from build123d import *

# Parameters (mm, degrees)
SKETCH1_W           = 50
SKETCH1_H           = 40
SKETCH1_W_2         = 44
SKETCH1_H_2         = 35.2
BOSS_EXTRUDE1_DEPTH = 5
SKETCH2_W           = 44
SKETCH2_H           = 35.2
BOSS_EXTRUDE2_DEPTH = 3
SKETCH3_R           = 6
BOSS_EXTRUDE3_DEPTH = 2
SKETCH4_R           = 1.6
CUT_EXTRUDE1_DEPTH  = 5
FILLET1_R           = 6
FILLET2_R           = 3
CUT_EXTRUDE2_DEPTH  = 3
SKETCH8_R           = 4
CUT_EXTRUDE3_DEPTH  = 3
CHAMFER1_SIZE       = 1
SKETCH9_W           = 3
SKETCH9_H           = 15
CUT_EXTRUDE4_DEPTH  = 2
FILLET3_R           = 2
BOSS_EXTRUDE5_START = 4
BOSS_EXTRUDE5_DEPTH = 4
SKETCH11_R          = 4
CUT_EXTRUDE5_DEPTH  = 4


with BuildPart() as part:
    # Sketch1 → Boss-Extrude1 (new body)
    with BuildSketch(Plane(origin=(0, 0, 0), x_dir=(1, 0, 0), z_dir=(0, 1, 0))):
        Rectangle(SKETCH1_W, SKETCH1_H)
        Rectangle(SKETCH1_W_2, SKETCH1_H_2, mode=Mode.SUBTRACT)
    extrude(amount=BOSS_EXTRUDE1_DEPTH)

    # Sketch2 → Boss-Extrude2 (add)
    with BuildSketch(Plane(origin=(0, 0, 0), x_dir=(-1, 0, 0), z_dir=(0, -1, 0))):
        Rectangle(SKETCH2_W, SKETCH2_H)
    extrude(amount=-BOSS_EXTRUDE2_DEPTH)

    # Sketch3 → Boss-Extrude3 (add)
    with BuildSketch(Plane(origin=(0, 3, 0), x_dir=(1, 0, 0), z_dir=(0, 1, 0))):
        with Locations(Location((7, 0, 0), (0, 0, 270))):
            Circle(SKETCH3_R)
    extrude(amount=BOSS_EXTRUDE3_DEPTH)

    # Sketch4 → Cut-Extrude1 (cut)
    with BuildSketch(Plane(origin=(0, 5, 0), x_dir=(1, 0, 0), z_dir=(0, 1, 0))):
        with Locations(Location((7, 0, 0), (0, 0, 270))):
            Circle(SKETCH4_R)
    extrude(amount=-CUT_EXTRUDE1_DEPTH, mode=Mode.SUBTRACT)

    # Fillet1
    fillet1_edges = [part.edges().sort_by_distance(p)[0] for p in [
        (22, 4, 17.6),
        (22, 4, -17.6),
        (-22, 4, -17.6),
        (-22, 4, 17.6),
        (-25, 2.5, -20),
        (25, 2.5, -20),
        (25, 2.5, 20),
        (-25, 2.5, 20),
    ]]
    fillet(fillet1_edges, radius=FILLET1_R)

    # Fillet2
    fillet2_edges = [part.edges().sort_by_distance(p)[0] for p in [
        (-25, 0, 0),
        (0, 0, -20),
        (25, 0, 0),
        (0, 0, 20),
        (23.242640687, 0, -18.242640687),
        (23.242640687, 0, 18.242640687),
        (-23.242640687, 0, 18.242640687),
        (-23.242640687, 0, -18.242640687),
    ]]
    fillet(fillet2_edges, radius=FILLET2_R)

    # Sketch6 → Cut-Extrude2 (cut)
    with BuildSketch(Plane(origin=(0, 0, 0), x_dir=(-1, 0, 0), z_dir=(0, -1, 0))):
        Polygon((-3.75, 0), (-5.375, 2.814582562), (-8.625, 2.814582562), (-10.25, 0), (-8.625, -2.814582562), (-5.375, -2.814582562), align=None)
    extrude(amount=-CUT_EXTRUDE2_DEPTH, mode=Mode.SUBTRACT)

    # Sketch8 → Cut-Extrude3 (cut)
    with BuildSketch(Plane(origin=(0, 0, 0), x_dir=(-1, 0, 0), z_dir=(0, -1, 0))):
        with Locations(Location((-12, -10, 0), (0, 0, 90))):
            Circle(SKETCH8_R)
        with Locations(Location((-12, 10, 0), (0, 0, 90))):
            Circle(SKETCH8_R)
    extrude(amount=-CUT_EXTRUDE3_DEPTH, mode=Mode.SUBTRACT)

    # Chamfer1
    chamfer1_edges = [part.edges().sort_by_distance(p)[0] for p in [
        (12, 0, 14),
        (12, 0, -6),
    ]]
    chamfer(chamfer1_edges, length=CHAMFER1_SIZE)

    # Sketch9 → Cut-Extrude4 (cut)
    with BuildSketch(Plane(origin=(0, 5, 0), x_dir=(1, 0, 0), z_dir=(0, 1, 0))):
        with Locations((23.5, 0)):
            Rectangle(SKETCH9_W, SKETCH9_H)
    extrude(amount=-CUT_EXTRUDE4_DEPTH, mode=Mode.SUBTRACT)

    # Fillet3
    fillet3_edges = [part.edges().sort_by_distance(p)[0] for p in [
        (23.5, 3, -7.5),
        (23.5, 3, 7.5),
    ]]
    fillet(fillet3_edges, radius=FILLET3_R - 0.0001)  # a hair under: the kernel refuses the full size

    # Sketch10 → Boss-Extrude5 (add)
    with BuildSketch(Plane(origin=(0, 3, 0), x_dir=(1, 0, 0), z_dir=(0, 1, 0)).offset(BOSS_EXTRUDE5_START)):
        with BuildLine():
            Line((-16, -17.6), (-16, -11.6))
            Line((-16, -11.6), (-22, -11.6))
            ThreePointArc((-22, -11.6), (-20.242640687, -15.842640687), (-16, -17.6))
        make_face()
        with BuildLine():
            Line((-16, 17.6), (-16, 11.6))
            Line((-16, 11.6), (-22, 11.6))
            ThreePointArc((-22, 11.6), (-20.242640687, 15.842640687), (-16, 17.6))
        make_face()
        with BuildLine():
            Line((16, 17.6), (16, 11.6))
            Line((16, 11.6), (22, 11.6))
            ThreePointArc((22, 11.6), (20.242640687, 15.842640687), (16, 17.6))
        make_face()
        with BuildLine():
            Line((22, -11.6), (16, -11.6))
            Line((16, -11.6), (16, -17.6))
            ThreePointArc((16, -17.6), (20.242640687, -15.842640687), (22, -11.6))
        make_face()
    extrude(amount=-BOSS_EXTRUDE5_DEPTH)

    # Sketch11 → Cut-Extrude5 (cut)
    with BuildSketch(Plane(origin=(0, 7, 0), x_dir=(1, 0, 0), z_dir=(0, 1, 0))):
        with Locations((16, 11.6)):
            Circle(SKETCH11_R)
        with Locations((16, -11.6)):
            Circle(SKETCH11_R)
        with Locations((-16, -11.6)):
            Circle(SKETCH11_R)
        with Locations((-16, 11.6)):
            Circle(SKETCH11_R)
    extrude(amount=-CUT_EXTRUDE5_DEPTH, mode=Mode.SUBTRACT)


solid = part.part
Can you work these out from the model? Positions are in its coordinate system, mm. A direction names the side the tool comes from. Give positions to 0.01 mm unless a question says otherwise; leave off trailing zeros. Loops run counter-clockwise (first coordinate to the right, second up) from the corner with the lowest first, then second, coordinate; pieces in that order, holes last. Notation, with made-up numbers: M 51.5,70.5 L 90.5,70.5 A24 cw 90.5,84.5 Z; hole C 9,46.5 d7. An arc over 180 degrees is marked long. One line per item, written item: value. Start each with the question number.
1) If we section it at A-A, the plane z = 10: Write out the boundary of the cut face in (x, y).
2) If we section it at C-C, the plane x = 12: Write out the boundary of the cut face in (y, z).
3) On a 3-axis mill with a long thin cutter (end or side, diameter ignored), from which of +Z, -Z, +X, -X, +Y, -Y can I reach the whole of each face in a straight line? I mean faces 1 (the face through (22, 4, 9)), 2 (the face through (5.6, 3, -1.3)), 3 (the face through (-20.289, 6.014, 15.796)). Say none if no direction works.
4) If we section it at B-B, the plane y = 5.75: Write out the boundary of the cut face in (x, z).
5) If we section it at D-D, the plane x = -11: Write out the boundary of the cut face in (y, z).
6) I'm going to push flat-ended pins straight in: pin 1 (2 mm diameter, centred on y = 4.5, z = -17, fed in from -X); pin 2 (3 mm diameter, centred on x = 7, z = -0.5, fed in from -Y); pin 3 (6 mm diameter, centred on x = 4, z = -2.5, fed in from +Y). Where does each tip first touch, or does it pass through?
7) If I drill on line 1 (X direction, y = 3.75, z = 0); line 2 (Z direction, x = 10.5, y = 4.25); line 3 (Y direction, x = -15.5, z = -16), over which ranges is the centre line in solid material (lowest first)? Write a range as [from, to].
8) Thinking about a two-plate mould opening in X: for faces 4 (the face through (-19, 7, -15)), 5 (the face through (-20.289, 6.014, -15.796)), 6 (the face through (7, 1, -2.815)), 7 (the face through (14.7, 1.99, -7.05)), which applies, +X half, -X half, draft (parallel to the pull), parting line (faces both ways), or undercut?
Completed:
1. outline: M -25,3 A3 ccw -22,0 L 7,0 L 8,1 L 8,3 L -22,3 L -22,5 L -25,5 Z; M 16,1 L 17,0 L 22,0 A3 ccw 25,3 L 25,5 L 22,5 L 22,3 L 16,3 Z
2. outline: M 0,-17 A3 ccw 3,-20 L 5,-20 L 5,-17.6 L 3,-17.6 L 3,-14 L 1,-14 L 0,-15 Z; M 0,-5 L 1,-6 L 3,-6 L 3,-3.32 L 5,-3.32 L 5,3.32 L 3,3.32 L 3,6 L 1,6 L 0,5 Z; M 0,15 L 1,14 L 3,14 L 3,17.6 L 5,17.6 L 5,20 L 3,20 A3 ccw 0,17 Z
3. face 1: +Y
3. face 2: -Y
3. face 3: +Z, -X, +Y
4. outline: M -22,-11.6 A6 ccw -16,-17.6 L -16,-15.6 A4 cw -20,-11.6 Z; M -22,11.6 L -20,11.6 A4 cw -16,15.6 L -16,17.6 A6 ccw Z; M 16,-17.6 A6 ccw 22,-11.6 L 20,-11.6 A4 cw 16,-15.6 Z; M 16,15.6 A4 cw 20,11.6 L 22,11.6 A6 ccw 16,17.6 Z
5. outline: M 0,-17 A3 ccw 3,-20 L 5,-20 L 5,-17.6 L 3,-17.6 L 3,17.6 L 5,17.6 L 5,20 L 3,20 A3 ccw 0,17 Z
6. pin 1: stops at x = -24.66
6. pin 2: stops at y = 3
6. pin 3: stops at y = 5
7. line 1: x = [-25, -22], [1, 5.4], [8.6, 13]
7. line 2: z = [-20, -17.6], [-4.87, 4.87], [17.6, 20]
7. line 3: y = [0, 3]
8. face 4: draft
8. face 5: -X half
8. face 6: undercut
8. face 7: undercut
